Autodesk Inventor part; units mm, degrees
ref_plane "YZ Plane" through (0, 0, 0) normal (1, 0, 0) x (0, 1, 0)
ref_plane "XZ Plane" through (0, 0, 0) normal (0, 1, 0) x (-1, 0, 0)
ref_plane "XY Plane" through (0, 0, 0) normal (0, 0, 1) x (1, 0, 0)
sketch "スケッチ1" plane through (0, 0, 0) normal (0, 1, 0) x (-1, 0, 0)
  arc A0 (209.8798, -23.6971) -> (38.3003, 12.1023) centre (-36.3979, -774.9853) ccw
  arc A1 (99.4686, -35.9265) -> (209.8798, -23.6971) centre (88.5018, 567.6156) ccw
  arc A2 (73.7238, -35.6322) -> (99.4686, -35.9265) centre (91.566, 398.982) ccw
  arc A3 (26.4399, -27.2272) -> (73.7238, -35.6322) centre (81.048, 142.776) ccw
  arc A4 (-0.8557, -13.8205) -> (26.4399, -27.2272) centre (58.458, 72.45) ccw
  arc A5 (-8.6045, -6.2961) -> (-0.8557, -13.8205) centre (17.4, 12.732) ccw
  arc A6 (-1.8835, 10.4943) -> (-8.6045, -6.2961) centre (0, 0) ccw
  arc A7 (18.284, 12.3227) -> (-1.8835, 10.4943) centre (18.66, -103.968) ccw
  arc A8 (38.3003, 12.1023) -> (18.284, 12.3227) centre (20.556, -690.396) ccw
extrude "押し出し1" add sketch "スケッチ1" along normal blind 4
sketch "スケッチ2" plane through (0, 0, 0) normal (0, -1, 0) x (1, 0, 0)
  circle A0 centre (-20, -2.2582) radius 5
  circle A1 centre (-130, -14.678) radius 5
  line L0 (0, 0) -> (-209.8798, -23.6971)
  dimension "d3" = 10
  dimension "d4" = 10
  dimension "d5" = 20
  dimension "d6" = 130
extrude "押し出し2" cut sketch "スケッチ2" against normal through all
equation "\"d4\" = d3"
properties part number "plate" material "木材 (オーク)"
Geometry: final body of the model. Coordinates: model frame, mm. Round coordinates to 2 decimals unless told otherwise and drop trailing zeros. Order: outer loops, then holes, each group sorted by start corner. A loop starts at its lowest first (then second) coordinate and runs counter-clockwise, first axis right, second up. Notation, with made-up numbers: (41, 37) -> (60, 37) arc R26 cw to (60, 59) -> close; hole circle Ø5 at (22, 62.25). An arc over 180 degrees is marked (long way). Put each result on its own line as item: value. Start each with the question number.
Q1. Section A-A on x = -22. Return the cut outline in (y, z), and give its area (3 significant figures).
Q2. Pull-direction query (Z, two-part tool) for faces 1 (the cylindrical face through (-125.38, 1.97, -16.59)), 2 (the cylindrical face through (-12.49, 1.97, -21.61)), 3 (the cylindrical face through (-8.019, 1.972, 11.835)), 4 (the cylindrical face through (-24.995, 1.972, -2.038)); classes: +Z half, -Z half, draft (parallel to the pull), parting line (faces both ways), or undercut.
Q3. Section B-B on z = -17. Return the cut outline in (x, y), and give its area (3 significant figures).
Q4. Section C-C on y = 0.7. Return the cut outline in (x, z).
Q5. Line query: probe 1 along Z at (x, y) = (-130, 2.15); probe 2 along Z at (x, y) = (-20, 3.1); probe 3 along Z at (x, y) = (-90, 2.9). Output: solid intervals per line, ascending.
Q6. Section D-D on x = -50. Return the cut outline in (y, z), and give its area (3 significant figures).
Q7. First-contact query: pin 1 (1.5 mm diameter, centred on y = 2.5, z = -25, fed in from +X); pin 2 (1.5 mm diameter, centred on x = -155, y = 3.5, fed in from +Z); pin 3 (2 mm diameter, centred on x = -157.5, y = 2, fed in from +Z). Flat tips, straight axial feed; report the tip coordinate or a pass-through.
Ans:
1. outline: (0, -25.69) -> (4, -25.69) -> (4, -6.84) -> (0, -6.84) -> close; (0, 2.32) -> (4, 2.32) -> (4, 12.32) -> (0, 12.32) -> close
1. area: 115 mm2
2. face 1: undercut
2. face 2: -Z half
2. face 3: +Z half
2. face 4: undercut
3. outline: (-188.42, 0) -> (-134.43, 0) -> (-134.43, 4) -> (-188.42, 4) -> close; (-125.57, 0) -> (-4.06, 0) -> (-4.06, 4) -> (-125.57, 4) -> close
3. area: 702 mm2
4. outline: (-209.88, -23.7) arc R603.64 ccw to (-99.47, -35.93) arc R434.99 ccw to (-73.72, -35.63) arc R178.56 ccw to (-26.44, -27.23) arc R104.69 ccw to (0.86, -13.82) arc R32.22 ccw to (8.6, -6.3) arc R10.66 ccw to (1.88, 10.49) arc R116.28 ccw to (-18.28, 12.32) arc R702.76 ccw to (-38.3, 12.1) arc R790.63 ccw to start; hole circle Ø10 at (-130, -14.68); hole circle Ø10 at (-20, -2.26)
5. probe 1: z = -34.6 to -19.68, -9.68 to -2.07
5. probe 2: z = -24.92 to -7.26, 2.74 to 12.33
5. probe 3: z = -36 to 5.47
6. outline: (0, -33.06) -> (4, -33.06) -> (4, 10.9) -> (0, 10.9) -> close
6. area: 176 mm2
7. pin 1: stops at x = -18.34
7. pin 2: stops at z = -7.69
7. pin 3: stops at z = -8.25
